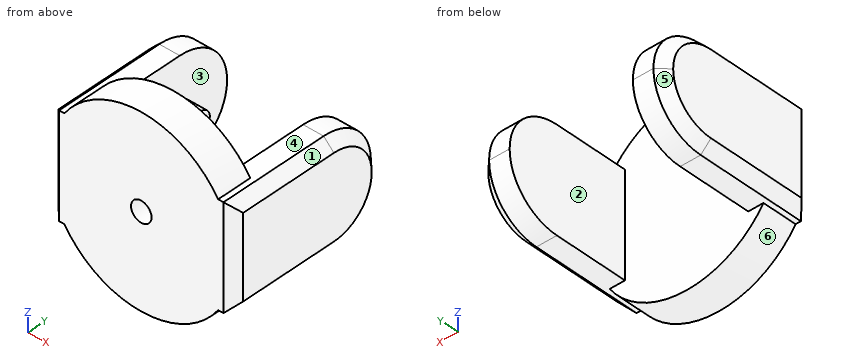
```python
from build123d import *

# Parameters (mm, degrees)
SKETCH1_R           = 45
BOSS_EXTRUDE1_DEPTH = 17
SKETCH2_W           = 50
SKETCH2_H           = 78
BOSS_EXTRUDE2_DEPTH = 15
SKETCH3_W           = 50
SKETCH3_H           = 78
BOSS_EXTRUDE3_DEPTH = 15
FILLET1_R           = 25
CHAMFER1_SIZE       = 5
SKETCH4_R           = 5
BOSS_EXTRUDE4_DEPTH = 10
SKETCH5_R           = 5
CUT_EXTRUDE1_DEPTH  = 10


# Some blends are built 0.0001 mm under size
with BuildPart() as part:
    # Sketch1 → Boss-Extrude1 (new body)
    with BuildSketch(Plane(origin=(0, 0, 0), x_dir=(1, 0, 0), z_dir=(0, 1, 0))):
        with Locations(Location((0, 0, 0), (0, 0, 270))):
            Circle(SKETCH1_R)
    extrude(amount=BOSS_EXTRUDE1_DEPTH)

    # Sketch2 → Boss-Extrude2 (add)
    with BuildSketch(Plane(origin=(45, 0, 0), x_dir=(0, 0, -1), z_dir=(1, 0, 0))):
        with Locations((0, 39)):
            Rectangle(SKETCH2_W, SKETCH2_H)
    extrude(amount=-BOSS_EXTRUDE2_DEPTH)

    # Sketch3 → Boss-Extrude3 (add)
    with BuildSketch(Plane(origin=(-45, 0, 0), x_dir=(0, 0, -1), z_dir=(1, 0, 0))):
        with Locations((0, 39)):
            Rectangle(SKETCH3_W, SKETCH3_H)
    extrude(amount=BOSS_EXTRUDE3_DEPTH)

    # Fillet1
    fillet1_edges = [part.edges().sort_by_distance(p)[0] for p in [
        (37.5, 78, -25),
        (37.5, 78, 25),
        (-37.5, 78, 25),
        (-37.5, 78, -25),
    ]]
    fillet(fillet1_edges, radius=FILLET1_R - 0.0001)  # a hair under: the kernel refuses the full size

    # Chamfer1
    # the kernel refuses this chamfer: 5 mm, written as the material it takes off along each edge
    with BuildSketch(Plane(origin=(45, 0, 5.6e-08), x_dir=(-0.9996219169112968, -0.027495876610585467, 0), z_dir=(0, 0, -1))) as chamfer1_piece_1:
        Polygon((CHAMFER1_SIZE * 0.999621916911, CHAMFER1_SIZE * 0.0274958766106), (-CHAMFER1_SIZE * 0.0274958766106, CHAMFER1_SIZE * 0.999621916911), (0, 0), align=None)
    chamfer1_piece_1_solid = extrude(amount=37.858414995, mode=Mode.PRIVATE)
    with BuildSketch(Plane(origin=(45, -12.85841494, -25), x_dir=(-0.9996219169112968, 0, -0.027495876610586317), z_dir=(0, 1, 0)), Plane(origin=(45, 53.0001, 25), x_dir=(-0.9996219169112968, 0, 0.027495876610586317), z_dir=(0, -1, 0)), Plane(origin=(-45, 53.0001, 25), x_dir=(-0.027495876610586317, 0, -0.9996219169112968), z_dir=(0, -1, 0))) as chamfer1_piece_2:
        Polygon((CHAMFER1_SIZE * 0.999621916911, CHAMFER1_SIZE * 0.0274958766106), (-CHAMFER1_SIZE * 0.0274958766106, CHAMFER1_SIZE * 0.999621916911), (0, 0), align=None)
    chamfer1_piece_2_solid = extrude(amount=65.85851494, mode=Mode.PRIVATE)
    with BuildSketch(Plane(origin=(-45, 0, 37.85841494), x_dir=(-0.027495876610586317, 0.9996219169112968, 0), z_dir=(0, 0, -1))) as chamfer1_piece_3:
        Polygon((CHAMFER1_SIZE * 0.999621916911, CHAMFER1_SIZE * 0.0274958766106), (-CHAMFER1_SIZE * 0.0274958766106, CHAMFER1_SIZE * 0.999621916911), (0, 0), align=None)
    chamfer1_piece_3_solid = extrude(amount=37.85841513, mode=Mode.PRIVATE)
    with BuildSketch(Plane(origin=(-45, -12.85841494, -25), x_dir=(0.9996219169112968, 0, -0.027495876610586317), z_dir=(0, 1, 0))) as chamfer1_piece_4:
        Polygon((CHAMFER1_SIZE * 0.999621916911, -CHAMFER1_SIZE * 0.0274958766106), (-CHAMFER1_SIZE * 0.0274958766106, -CHAMFER1_SIZE * 0.999621916911), (0, 0), align=None)
    chamfer1_piece_4_solid = extrude(amount=65.85851494, mode=Mode.PRIVATE)
    with BuildSketch(Plane(origin=(45, 53.0001, 0.0001), x_dir=(0, 0, 1), z_dir=(0, -1, 0))) as chamfer1_piece_5:
        Polygon((24.9999 - CHAMFER1_SIZE, 0), (24.9999, CHAMFER1_SIZE), (24.9999, 0), align=None)
    chamfer1_piece_5_solid = revolve(axis=Axis((45, 53.0001, 0.0001), (-1, 0, 0)), revolution_arc=90, mode=Mode.PRIVATE)
    with BuildSketch(Plane(origin=(45, 53.0001, -0.0001), x_dir=(0, 0, -1), z_dir=(0, -1, 0))) as chamfer1_piece_6:
        Polygon((24.9999 - CHAMFER1_SIZE, 0), (24.9999, -CHAMFER1_SIZE), (24.9999, 0), align=None)
    chamfer1_piece_6_solid = revolve(axis=Axis((45, 53.0001, -0.0001), (1, 0, 0)), revolution_arc=90, mode=Mode.PRIVATE)
    with BuildSketch(Plane(origin=(-45, 53.0001, -0.0001), x_dir=(0, 0, -1), z_dir=(0, -1, 0))) as chamfer1_piece_7:
        Polygon((24.9999 - CHAMFER1_SIZE, 0), (24.9999, CHAMFER1_SIZE), (24.9999, 0), align=None)
    chamfer1_piece_7_solid = revolve(axis=Axis((-45, 53.0001, -0.0001), (1, 0, 0)), revolution_arc=90, mode=Mode.PRIVATE)
    with BuildSketch(Plane(origin=(-45, 53.0001, 0.0001), x_dir=(0, 1, 0), z_dir=(0, 0, -1))) as chamfer1_piece_8:
        Polygon((24.9999 - CHAMFER1_SIZE, 0), (24.9999, CHAMFER1_SIZE), (24.9999, 0), align=None)
    chamfer1_piece_8_solid = revolve(axis=Axis((-45, 53.0001, 0.0001), (1, 0, 0)), revolution_arc=90, mode=Mode.PRIVATE)
    with BuildSketch(Plane(origin=(-45, 78, -0.0001), x_dir=(-0.027495876610586282, -0.9996219169112968, 0), z_dir=(0, 0, 1))) as chamfer1_piece_9:
        Polygon((CHAMFER1_SIZE * 0.999621916911, CHAMFER1_SIZE * 0.0274958766106), (-CHAMFER1_SIZE * 0.0274958766106, CHAMFER1_SIZE * 0.999621916911), (0, 0), align=None)
    chamfer1_piece_9_solid = extrude(amount=0.0002, mode=Mode.PRIVATE)
    with BuildSketch(Plane(origin=(45, 78, -0.0001), x_dir=(0.027495876610586282, -0.9996219169112968, 0), z_dir=(0, 0, 1))) as chamfer1_piece_10:
        Polygon((CHAMFER1_SIZE * 0.999621916911, -CHAMFER1_SIZE * 0.0274958766106), (-CHAMFER1_SIZE * 0.0274958766106, -CHAMFER1_SIZE * 0.999621916911), (0, 0), align=None)
    chamfer1_piece_10_solid = extrude(amount=0.0002, mode=Mode.PRIVATE)
    with BuildSketch(Plane(origin=(-45, 0, -1.91e-07), x_dir=(-0.027495876610586334, 0.9996219169112968, 0), z_dir=(0, 0, -1))) as chamfer1_piece_11:
        Polygon((CHAMFER1_SIZE * 0.999621916911, CHAMFER1_SIZE * 0.0274958766106), (-CHAMFER1_SIZE * 0.0274958766106, CHAMFER1_SIZE * 0.999621916911), (0, 0), align=None)
    chamfer1_piece_11_solid = extrude(amount=37.858414749, mode=Mode.PRIVATE)
    with BuildSketch(Plane(origin=(45, 0, 37.85841494), x_dir=(-0.9996219169112968, -0.027495876610586372, 0), z_dir=(0, 0, -1))) as chamfer1_piece_12:
        Polygon((CHAMFER1_SIZE * 0.999621916911, CHAMFER1_SIZE * 0.0274958766106), (-CHAMFER1_SIZE * 0.0274958766106, CHAMFER1_SIZE * 0.999621916911), (0, 0), align=None)
    chamfer1_piece_12_solid = extrude(amount=37.858414884, mode=Mode.PRIVATE)
    add([chamfer1_piece_1_solid, chamfer1_piece_2_solid, chamfer1_piece_3_solid, chamfer1_piece_4_solid, chamfer1_piece_5_solid, chamfer1_piece_6_solid, chamfer1_piece_7_solid, chamfer1_piece_8_solid, chamfer1_piece_9_solid, chamfer1_piece_10_solid, chamfer1_piece_11_solid, chamfer1_piece_12_solid], mode=Mode.SUBTRACT)

    # Sketch4 → Boss-Extrude4 (add)
    with BuildSketch(Plane(origin=(-30, 0, 0), x_dir=(0, 0, -1), z_dir=(1, 0, 0))):
        with Locations(Location((0, 53, 0), (0, 0, 180))):
            Circle(SKETCH4_R)
    extrude(amount=BOSS_EXTRUDE4_DEPTH)

    # Sketch5 → Cut-Extrude1 (cut)
    with BuildSketch(Plane(origin=(0, 0, 0), x_dir=(-1, 0, 0), z_dir=(0, -1, 0))):
        with Locations(Location((0, 0, 0), (0, 0, 90))):
            Circle(SKETCH5_R)
    extrude(amount=-CUT_EXTRUDE1_DEPTH, mode=Mode.SUBTRACT)


solid = part.part
```
Here's how the part is built. I have some questions about the finished solid (model axes, mm). Face numbers are marked on the shaded views. A direction names the side the tool comes from. Give positions to 0.01 mm unless a question says otherwise; leave off trailing zeros. Loops run counter-clockwise (first coordinate to the right, second up) from the corner with the lowest first, then second, coordinate; pieces in that order, holes last. Notation, with made-up numbers: M -19.75,0 L 21.25,0 A22 cw 21.25,26 Z; hole C 34,-9 d5. An arc over 180 degrees is marked long. Return JSON: item names as keys, results as strings.
Item 1: Thinking about a two-plate mould opening in X: for the marked faces 3, 4, 5 and 6, which applies, released by +X, released by -X, zero draft, split by the parting line, or undercut?
A:
{"face 3": "undercut", "face 4": "zero draft", "face 5": "released by -X", "face 6": "split by the parting line"}
Item 2: Imagine slicing it at C-C on z = -39. List the corners of the cut face in (x, y) for me.
A:
{"outline": "M -22.45,0 L 22.45,0 L 22.45,17 L -22.45,17 Z"}
Item 3: I'm going to push flat-ended pins straight in: pin 1 Ø2 at (x, z) = (0.5, 10.5) entering from +Y; pin 2 Ø3 at (x, y) = (2, 19.5) entering from -Z; pin 3 Ø5 at (x, y) = (37, 36.5) entering from -Z; pin 4 Ø3 at (x, y) = (-34, 28.5) entering from +Z. Where does each tip first touch, or does it pass through?
A:
{"pin 1": "stops at y = 17", "pin 2": "passes through", "pin 3": "stops at z = -25", "pin 4": "stops at z = 25"}
Item 4: Please list where these lines run through material, in increasing order: line 1 (X direction, y = 26, z = -13); line 2 (Z direction, x = -36, y = 51); line 3 (Y direction, x = -31, z = -32).
A:
{"line 1": "x = -45 to -30, 30 to 45", "line 2": "z = -25 to 25", "line 3": "y = 0 to 17"}
Item 5: On a 3-axis mill with a long thin cutter (end or side, diameter ignored), from which of +Z, -Z, +X, -X, +Y, -Y can I reach the whole of each face in a straight line? I mean the marked faces 1 and 2. Say none if no direction works.
A:
{"face 1": "+Z, +X, +Y, -Y", "face 2": "+Z, -Z, +Y"}
Item 6: Imagine slicing it at A-A on y = 35. List the corners of the cut face in (x, z) for me, then the cut area to 3 significant figures.
A:
{"outline": "M -45,-20 L -40,-25 L -30,-25 L -30,25 L -40,25 L -45,20 Z; M 30,-25 L 40,-25 L 45,-20 L 45,20 L 40,25 L 30,25 Z", "area": "1,450 mm^2"}
Item 7: Imagine slicing it at D-D on x = -3. List the corners of the cut face in (y, z) for me, then the cut area to 3 significant figures.
A:
{"outline": "M 0,-44.9 L 17,-44.9 L 17,44.9 L 0,44.9 L 0,4 L 10,4 L 10,-4 L 0,-4 Z", "area": "1,450 mm^2"}
